from build123d import *

# Parameters (mm, degrees)
F0_W        = 35.56
F0_H        = 31.75
F1_DEPTH    = 12.7
F2_R        = 5.08
F3_T1_DEPTH = 47.625
F3_T4_ANGLE = 90
F3_T6_ANGLE = 90
F4_R        = 5.08
F5_R        = 5.08


# Not quite as in the source:
# - a fillet or chamfer that OpenCascade refuses, or shapes differently, is made with other operations: its cross-section is extruded or revolved along the edge and cut away or added


with BuildPart() as f1:
    # F0 (on Front) → F1 (new body, symmetric)
    with BuildSketch(Plane.XZ):
        Rectangle(F0_W, F0_H)
    extrude(amount=F1_DEPTH, both=True)

    # F2
    f2_edges = [f1.edges().sort_by_distance(p)[0] for p in [
        (0, -12.7, 15.875),
        (0, 12.7, 15.875),
        (17.78, 0, 15.875),
    ]]
    fillet(f2_edges, radius=F2_R)

    # F3: fillet of radius 6.35 on 2 edges, made by hand

    # F3_s2 → F3_t1 (cut)
    with BuildSketch(Plane.XY.offset(-31.75)):
        with BuildLine():
            ThreePointArc((11.43, -12.7), (15.9201280605, -10.8401280605), (17.78, -6.35))
            Line((17.78, -6.35), (17.78, -12.7))
            Line((17.78, -12.7), (11.43, -12.7))
        make_face()
        with BuildLine():
            ThreePointArc((11.43, 12.7), (15.9201280605, 10.8401280605), (17.78, 6.35))
            Line((17.78, 6.35), (17.78, 12.7))
            Line((17.78, 12.7), (11.43, 12.7))
        make_face()
    extrude(amount=F3_T1_DEPTH, mode=Mode.SUBTRACT)

    # F3_s3 → F3_t4 (revolve, cut)
    with BuildSketch(Plane.XZ.offset(-6.35)):
        with BuildLine():
            ThreePointArc((12.7, 15.875), (16.2921024484, 14.3871024484), (17.78, 10.795))
            Line((17.78, 10.795), (17.78, 15.875))
            Line((17.78, 15.875), (12.7, 15.875))
        make_face()
    revolve(axis=Axis((11.43, 6.35, 15.875), (0, 0, 1)), revolution_arc=F3_T4_ANGLE, mode=Mode.SUBTRACT)

    # F3_s5 → F3_t6 (revolve, cut)
    with BuildSketch(Plane.YZ.offset(11.43)):
        with BuildLine():
            ThreePointArc((-7.62, 15.875), (-11.2121024484, 14.3871024484), (-12.7, 10.795))
            Line((-12.7, 10.795), (-12.7, 15.875))
            Line((-12.7, 15.875), (-7.62, 15.875))
        make_face()
    revolve(axis=Axis((11.43, -6.35, 15.875), (0, 0, 1)), revolution_arc=F3_T6_ANGLE, mode=Mode.SUBTRACT)

    # F4
    f4_edges = [f1.edges().sort_by_distance(p)[0] for p in [
        (-17.78, 0, -15.875),
    ]]
    fillet(f4_edges, radius=F4_R)

    # F5
    f5_edges = [f1.edges().sort_by_distance(p)[0] for p in [
        (-16.292102, -12.7, -14.387102),
        (-16.292102, 12.7, -14.387102),
    ]]
    fillet(f5_edges, radius=F5_R)


solid = f1.part
Geometry check sheet. Reference: the model listing, model coordinates, mm. Coordinates: 2 decimals unless noted, no trailing zeros. Order: outer loops, then holes, each group sorted by start corner. A loop starts at its lowest first (then second) coordinate and runs counter-clockwise, first axis right, second up. Notation, with made-up numbers: (-36, -19.5) - (-28, -19.5) arc R14 cw to (-28, 0.5) - close; hole circle Ø2 at (1, 69). An arc over 180 degrees is marked (long way). One line per item, written item: value.
(1) Sectioned sample at B-B (y = -1.5). Enter the section's corners in (x, z) (3 decimals).
Data:
outline: (-17.78, -10.795) arc R5.08 ccw to (-12.7, -15.875) - (12.7, -15.875) arc R5.08 ccw to (17.78, -10.795) - (17.78, 10.795) arc R5.08 ccw to (12.7, 15.875) - (-12.7, 15.875) arc R5.08 ccw to (-17.78, 10.795) - close
(2) Depth check by flat-ended pin: pin 1 Ø1.5 at (y, z) = (7.5, 12) entering from -X. Enter the tip coordinate at first touch or a pass-through.
Data:
pin 1: stops at x = -17.76
(3) Thickness scan on probe 1 along X at (y, z) = (11, 13); probe 2 along Y at (x, z) = (12, -5); probe 3 along Y at (x, z) = (14.5, 14.5). Record the ranges inside material, lowest first. Write a range as from..to.
Data:
probe 1: x = -15.79..14.97
probe 2: y = -12.67..12.67
probe 3: y = -9.97..9.97
(4) Sectioned sample at A-A (z = 8). Enter the section's corners in (x, y).
Data:
outline: (-17.78, -7.62) arc R5.08 ccw to (-12.7, -12.7) - (11.43, -12.7) arc R6.35 ccw to (17.78, -6.35) - (17.78, 6.35) arc R6.35 ccw to (11.43, 12.7) - (-12.7, 12.7) arc R5.08 ccw to (-17.78, 7.62) - close
